Check sheet for the drawn part. Datum: minimum x, y, z corner. Units: mm. A direction names the side the tool comes from. Give positions to 0.01 mm unless a question says otherwise; leave off trailing zeros. Write each loop counter-clockwise with the first axis right and the second up, starting at its lowest first coordinate (ties: lowest second). Pieces come first, ordered by that corner, then holes.
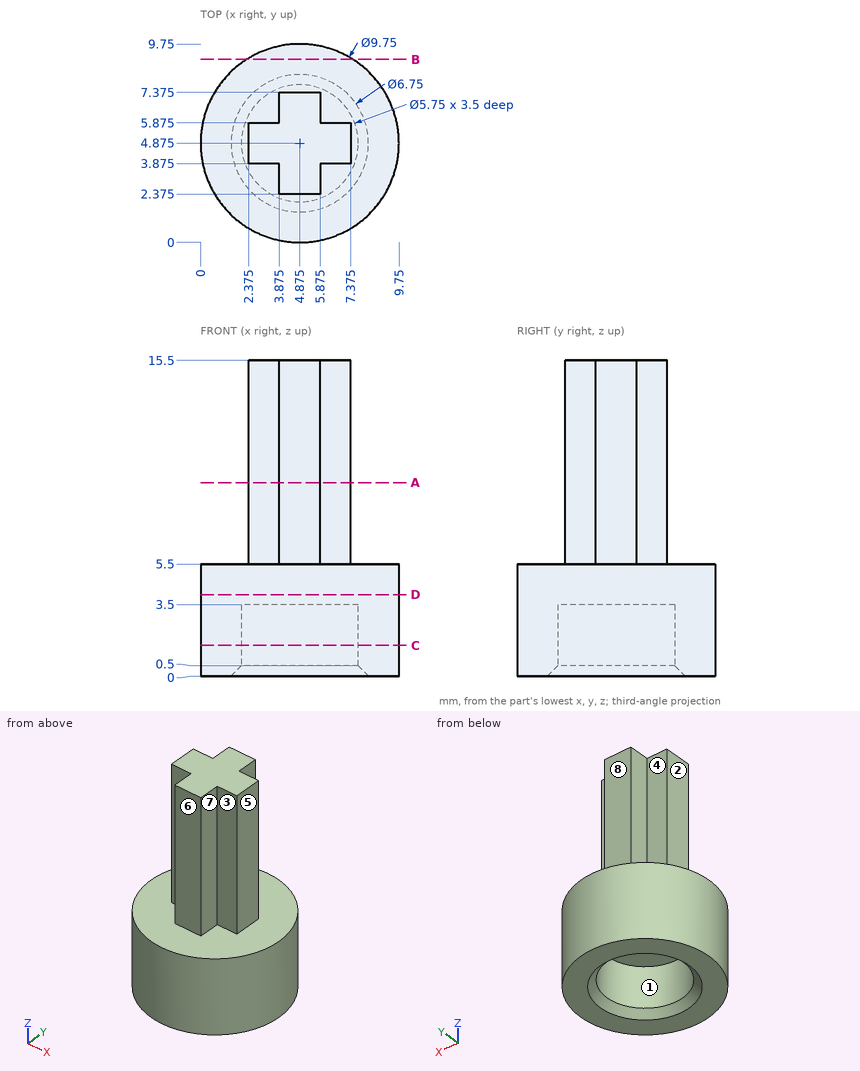
1) Access from +Z, -Z, +X, -X, +Y, -Y to the whole of each face (thin tool, end or side, straight path). Record for the marked faces 4, 5, 6, 7 and 8.
2) Gauge pin test, flat ends, axial feed: pin 1 (1.2 mm diameter, centred on x = 3, z = 10.5, fed in from -Y) (3 decimals); pin 2 (4 mm diameter, centred on x = 4, z = 2.5, fed in from -Y); pin 3 (1 mm diameter, centred on x = 4.5, z = 12.5, fed in from +Y) (3 decimals); pin 4 (0.8 mm diameter, centred on y = 6.5, z = 9.5, fed in from +X) (3 decimals). Record the tip position at first contact, or that the pin passes through.
3) Sectioned sample at C-C on z = 1.5. Record the boundary of the cut face in (x, y) (3 decimals), then the cut area to 3 significant figures.
4) Sectioned sample at A-A on z = 9.5. Record the boundary of the cut face in (x, y) (3 decimals), then the cut area to 3 significant figures.
5) Draft check along X on the marked faces 1, 2 and 3. Enter one of: +X half, -X half, draft (parallel to the pull), parting line (faces both ways), or undercut.
6) Sectioned sample at D-D on z = 4. Record the boundary of the cut face in (x, y) (3 decimals), then the cut area to 3 significant figures.
7) Sectioned sample at B-B on y = 9. Record the boundary of the cut face in (x, z), then the cut area to 3 significant figures.
8) Scan lines: L1, parallel to X at y = 6.75, z = 7.5 (3 decimals); L2, parallel to Z at x = 8.75, y = 5.5; L3, parallel to Y at x = 4.5, z = 8 (3 decimals). Record each from-to range of solid material in increasing order.
Answers below:
1. face 4: +Z, -X, +Y
1. face 5: +Z, +X, +Y, -Y
1. face 6: +Z, +X, -X, -Y
1. face 7: +Z, +X, -Y
1. face 8: +Z, +X, -X, +Y
2. pin 1: stops at y = 3.875
2. pin 2: stops at y = 0
2. pin 3: stops at y = 7.375
2. pin 4: stops at x = 5.875
3. outline: circle Ø9.75 at (4.875, 4.875); hole circle Ø5.75 at (4.875, 4.875)
3. area: 48.7 mm2
4. outline: (2.375, 3.875) - (3.875, 3.875) - (3.875, 2.375) - (5.875, 2.375) - (5.875, 3.875) - (7.375, 3.875) - (7.375, 5.875) - (5.875, 5.875) - (5.875, 7.375) - (3.875, 7.375) - (3.875, 5.875) - (2.375, 5.875) - close
4. area: 16.0 mm2
5. face 1: undercut
5. face 2: -X half
5. face 3: draft
6. outline: circle Ø9.75 at (4.875, 4.875)
6. area: 74.7 mm2
7. outline: (2.28, 0) - (7.47, 0) - (7.47, 5.5) - (2.28, 5.5) - close
7. area: 28.6 mm2
8. L1: x = 3.875 to 5.875
8. L2: z = 0 to 5.5
8. L3: y = 2.375 to 7.375
